from build123d import *

# Parameters (mm, degrees)
CROQUIS1_W              = 2.8
CROQUIS1_H              = 5.8
SALIENTE_EXTRUIR1_DEPTH = 1.5
REDONDEO1_R             = 2


with BuildPart() as part:
    # Croquis1 → Saliente-Extruir1 (new, symmetric)
    # profile 1 of 3: a face of its own
    with BuildSketch(Plane.XY):
        Polygon((-4.5, -2.5), (-4.5, -6.5), (-1.5, -6.5), (10.5, -6.5), (10.5, 6.5), (-1.5, 6.5), (-4.5, 6.5), (-4.5, 0.5), align=None)
        with Locations((4.1, 0)):
            Rectangle(CROQUIS1_W, CROQUIS1_H, mode=Mode.SUBTRACT)
    # profile 2 of 3: a face of its own
    with BuildSketch(Plane.XY):
        Polygon((-4.5, -2.5), (-4.5, -6.5), (-1.5, -6.5), (10.5, -6.5), (10.5, 6.5), (-1.5, 6.5), (-4.5, 6.5), (-4.5, 0.5), align=None)
        with Locations((4.1, 0)):
            Rectangle(CROQUIS1_W, CROQUIS1_H, mode=Mode.SUBTRACT)
    # profile 3 of 3: a face of its own
    with BuildSketch(Plane.XY):
        Polygon((-4.5, -2.5), (-4.5, -6.5), (-1.5, -6.5), (10.5, -6.5), (10.5, 6.5), (-1.5, 6.5), (-4.5, 6.5), (-4.5, 0.5), align=None)
        with Locations((4.1, 0)):
            Rectangle(CROQUIS1_W, CROQUIS1_H, mode=Mode.SUBTRACT)
    extrude(amount=SALIENTE_EXTRUIR1_DEPTH, both=True)

    # Redondeo1
    redondeo1_edges = [part.edges().sort_by_distance(p)[0] for p in [
        (10.5, 6.5, 0),
        (10.5, -6.5, 0),
    ]]
    fillet(redondeo1_edges, radius=REDONDEO1_R)


solid = part.part
For this review, take the finished solid that the model builds, in its own axes (mm). A direction names the side the tool comes from. Coordinates: 2 decimals unless noted, no trailing zeros. Loops run counter-clockwise (first coordinate to the right, second up) from the corner with the lowest first, then second, coordinate; pieces in that order, holes last. Notation, with made-up numbers: (-31.75, 70.5) - (-21.75, 70.5) arc R17 cw to (-21.75, 102.5) - close; hole circle Ø4 at (83.25, 44.25). An arc over 180 degrees is marked (long way). Return JSON: item names as keys, results as strings.
Item 1: For faces 1 (the flat face through (10.5, 0, 0)), 2 (the flat face through (4, -2.9, 0)), list the 3-axis set-ups (+Z, -Z, +X, -X, +Y, -Y) from which the entire face can be reached by the end or side of a thin tool; tool diameter is ignored.
Determined:
{"face 1": "+Z, -Z, +X, +Y, -Y", "face 2": "+Z, -Z"}
Item 2: Mouldability with a two-part tool opening along X and no side actions: class faces 3 (the cylindrical face through (9.9, 5.93, 0.02)), 4 (the flat face through (4, 2.9, 0)), 5 (the flat face through (1, 0, -1.5)), 6 (the flat face through (2.7, 0, 0)) as pulls with the +X half, pulls with the -X half, needs draft (parallel to the pull), parting line crosses it, or undercut.
Determined:
{"face 3": "pulls with the +X half", "face 4": "undercut", "face 5": "needs draft", "face 6": "undercut"}
Item 3: Take a section at C-C (z = 0). Give the boundary of the cut face in (x, y).
Determined:
{"outline": "(-4.5, -6.5) - (8.5, -6.5) arc R2 ccw to (10.5, -4.5) - (10.5, 4.5) arc R2 ccw to (8.5, 6.5) - (-4.5, 6.5) - close; hole (2.7, -2.9) - (5.5, -2.9) - (5.5, 2.9) - (2.7, 2.9) - close"}
Item 4: Take a section at B-B (x = 3). Give the boundary of the cut face in (y, z), then the cut area to 3 significant figures.
Determined:
{"outline": "(-6.5, -1.5) - (-2.9, -1.5) - (-2.9, 1.5) - (-6.5, 1.5) - close; (2.9, -1.5) - (6.5, -1.5) - (6.5, 1.5) - (2.9, 1.5) - close", "area": "21.6 mm2"}
Item 5: Take a section at A-A (y = 2.5). Give the boundary of the cut face in (x, z).
Determined:
{"outline": "(-4.5, -1.5) - (2.7, -1.5) - (2.7, 1.5) - (-4.5, 1.5) - close; (5.5, -1.5) - (10.5, -1.5) - (10.5, 1.5) - (5.5, 1.5) - close"}
Item 6: For line 1 (Y direction, x = 3.5, z = -1); line 2 (X direction, y = 0.25, z = 1.1); line 3 (Y direction, x = 9.5, z = -0.95), list the stretches that pass through material, from the lowest coordinate up.
Determined:
{"line 1": "y = -6.5 to -2.9, 2.9 to 6.5", "line 2": "x = -4.5 to 2.7, 5.5 to 10.5", "line 3": "y = -6.23 to 6.23"}
